CAD build for the part. Positions are in the model's coordinates, mm. A direction names the side the tool comes from. Round coordinates to 2 decimals unless told otherwise and drop trailing zeros. Order: outer loops, then holes, each group sorted by start corner. A loop starts at its lowest first (then second) coordinate and runs counter-clockwise, first axis right, second up. Notation, with made-up numbers: M 62.25,45 L 98.25,45 A29 ccw 98.25,78 Z; hole C 61.25,-22 d8. An arc over 180 degrees is marked long. Answer as a JSON object with one key per item and string values.
```python
from build123d import *

# Parameters (mm, degrees)
F0_W     = 30
F0_H     = 180
F0_R     = 10.01
F1_DEPTH = 10
F2_R     = 10.01
F3_DEPTH = 10
F5_DEPTH = 10


with BuildPart() as f1:
    # F0 (on Front) → F1 (new body)
    with BuildSketch(Plane.XZ):
        Rectangle(F0_W, F0_H)
        Circle(F0_R, mode=Mode.SUBTRACT)
    extrude(amount=F1_DEPTH)

    # F2 (on face) → F3 (join)
    with BuildSketch(Plane.XZ.offset(10)):
        with BuildLine():
            Line((-15, -20), (-15, 20))
            ThreePointArc((-15, 20), (-25, 0), (-15, -20))
        make_face()
        with BuildLine():
            Line((15, -20), (15, 20))
            ThreePointArc((15, 20), (0, 25), (-15, 20))
            Line((-15, 20), (-15, -20))
            ThreePointArc((-15, -20), (0, -25), (15, -20))
        make_face()
        Circle(F2_R, mode=Mode.SUBTRACT)
        with BuildLine():
            ThreePointArc((15, -20), (22.360679775, -11.1803398875), (25, 0))
            ThreePointArc((25, 0), (22.360679775, 11.1803398875), (15, 20))
            Line((15, 20), (15, -20))
        make_face()
    extrude(amount=-F3_DEPTH)

    # F4 (on face) → F5 (join)
    with BuildSketch(Plane.XZ.offset(10)):
        with BuildLine():
            Line((-15, -90), (-15, -47.5735931288))
            ThreePointArc((-15, -47.5735931288), (-25.9807621135, -126.7423461417), (45, -90))
            ThreePointArc((45, -90), (36.7423461417, -64.0192378865), (15, -47.5735931288))
            Line((15, -47.5735931288), (15, -90))
            Line((15, -90), (-15, -90))
        make_face()
        with BuildLine():
            ThreePointArc((15, -47.5735931288), (0, -45), (-15, -47.5735931288))
            Line((-15, -47.5735931288), (-15, -90))
            Line((-15, -90), (15, -90))
            Line((15, -90), (15, -47.5735931288))
        make_face()
        with BuildLine():
            ThreePointArc((15, 47.5735931288), (36.7423461417, 64.0192378865), (45, 90))
            ThreePointArc((45, 90), (-25.9807621135, 126.7423461417), (-15, 47.5735931288))
            Line((-15, 47.5735931288), (-15, 90))
            Line((-15, 90), (15, 90))
            Line((15, 90), (15, 47.5735931288))
        make_face()
        with BuildLine():
            Line((-15, 90), (-15, 47.5735931288))
            ThreePointArc((-15, 47.5735931288), (0, 45), (15, 47.5735931288))
            Line((15, 47.5735931288), (15, 90))
            Line((15, 90), (-15, 90))
        make_face()
    extrude(amount=-F5_DEPTH)


solid = f1.part
```
Item 1: Drop flat-ended pins along their axis: pin 1 Ø4 at (y, z) = (-2, 45) entering from +X; pin 2 Ø1 at (x, y) = (18, -1.5) entering from +Z; pin 3 Ø1 at (y, z) = (-3.5, 50.5) entering from +X; pin 4 Ø18 at (x, z) = (0, 0) entering from +Y. Give the stop position or say it passes through.
Worked answers:
{"pin 1": "stops at x = 15", "pin 2": "stops at z = 131.46", "pin 3": "stops at x = 22.45", "pin 4": "passes through"}
Item 2: Two-plate mould, pull along Z, no slides. Class faces 1 (the flat face through (-11, 0, 2)), 2 (the flat face through (-15, -5, -34)): released by +Z, released by -Z, zero draft, split by the parting line, or undercut.
Worked answers:
{"face 1": "zero draft", "face 2": "undercut"}
Item 3: 3-axis set-ups, long thin cutter, end or side, ignore diameter. For faces 3 (the cylindrical face through (-7.944, -4.93, -6.091)), 4 (the flat face through (15, -5, -34)), 5 (the flat face through (-15, -5, 34)): which of +Z, -Z, +X, -X, +Y, -Y reach the whole face in a straight line?
Worked answers:
{"face 3": "+Y, -Y", "face 4": "+X, +Y, -Y", "face 5": "-X, +Y, -Y"}
Item 4: Saw through at C-C on y = -7. List the corners of the cut face in (x, z), and give its area (3 significant figures).
Worked answers:
{"outline": "M -15,-47.57 A45 ccw long 15,-47.57 L 15,-20 A25 ccw 15,20 L 15,47.57 A45 ccw long -15,47.57 L -15,20 A25 ccw -15,-20 Z; hole C 0,0 d20.02", "area": "15,700 mm2"}
Item 5: Wall check: line 1 along Z through (x, y) = (0, -6.5); line 2 along Z through (x, y) = (17, -2.5); line 3 along Z through (x, y) = (-19.5, -4.25). Give the ranges that are in metal, low to high. Write a range as [from, to].
Worked answers:
{"line 1": "z = [-135, -10.01], [10.01, 135]", "line 2": "z = [-131.67, -48.33], [-18.33, 18.33], [48.33, 131.67]", "line 3": "z = [-130.56, -49.44], [-15.64, 15.64], [49.44, 130.56]"}
Item 6: Saw through at B-B on x = 0. List the corners of the cut face in (y, z).
Worked answers:
{"outline": "M -10,-135 L 0,-135 L 0,-10.01 L -10,-10.01 Z; M -10,10.01 L 0,10.01 L 0,135 L -10,135 Z"}
Item 7: Saw through at A-A on z = 0. List the corners of the cut face in (x, y).
Worked answers:
{"outline": "M -25,-10 L -10.01,-10 L -10.01,0 L -25,0 Z; M 10.01,-10 L 25,-10 L 25,0 L 10.01,0 Z"}
Item 8: Saw through at D-D on z = -53. List the corners of the cut face in (x, y).
Worked answers:
{"outline": "M -25.61,-10 L 25.61,-10 L 25.61,0 L -25.61,0 Z"}
